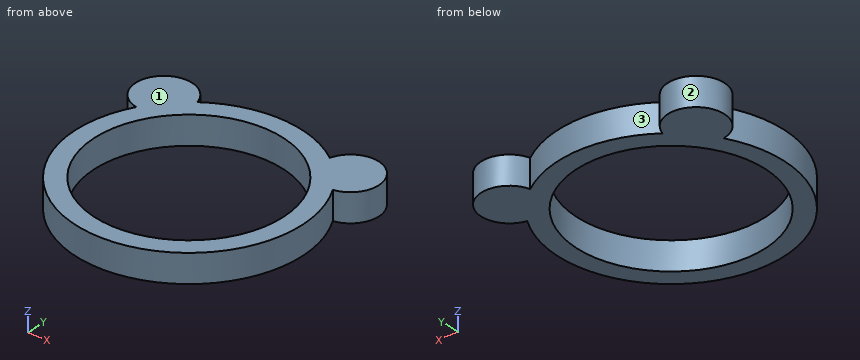
from build123d import *

# Parameters (mm, degrees)
CYLINDER002_R               = 10
CYLINDER002_DEPTH           = 10
CYLINDER001_R               = 3
CYLINDER001_DEPTH           = 3
CYLINDER001_PLACEMENT_ANGLE = 45
CYLINDER_R                  = 12
CYLINDER_DEPTH              = 3


with BuildPart() as hole:
    # Cylinder002 → Cylinder002 (new body)
    with BuildSketch(Plane.XY.offset(-4)):
        Circle(CYLINDER002_R)
    extrude(amount=CYLINDER002_DEPTH)


with BuildPart() as left_ear:
    # Cylinder001 → Cylinder001 (new body)
    with BuildSketch(Plane.XY):
        Circle(CYLINDER001_R)
    extrude(amount=CYLINDER001_DEPTH)


with BuildPart() as left_ear_1:
    # Cylinder001 placement: moved
    add(left_ear.part.moved(Location((-9.899495, 8.899495, 0))).rotate(Axis((-9.899495, 8.899495, 0), (0, 0, 1)), CYLINDER001_PLACEMENT_ANGLE))


with BuildPart() as right_ear:
    # Part__Mirroring: instance of left-ear
    add(left_ear_1.part.mirror(Plane(origin=(0, 0, 0), x_dir=(0, -1, 0), z_dir=(1, 0, 0))))


with BuildPart() as base_cylinder:
    # Cylinder → Cylinder (new body)
    with BuildSketch(Plane.XY):
        Circle(CYLINDER_R)
    extrude(amount=CYLINDER_DEPTH)


with BuildPart() as ring_with_ears:
    # Fusion base: copy of left-ear
    add(left_ear_1.part)

    # Fusion: union right-ear, base-cylinder
    add(right_ear.part)
    add(base_cylinder.part)

    # Cut: cut hole
    add(hole.part, mode=Mode.SUBTRACT)


solid = ring_with_ears.part
Source: CAD feature listing. Evaluate the final solid. Frame: model axes, mm. Face numbers are marked on the shaded views. Give positions to 0.01 mm unless a question says otherwise; leave off trailing zeros. Write each loop counter-clockwise with the first axis right and the second up, starting at its lowest first coordinate (ties: lowest second). Pieces come first, ordered by that corner, then holes. Notation, with made-up numbers: M 33,-20 L 92,-20 A7 cw 92,-16 Z; hole C 13,29 d6. An arc over 180 degrees is marked long. Return JSON: item names as keys, results as strings. Group by question number.
1) Pull-direction query (X, two-part tool) for the marked faces 1, 2 and 3; classes: pulls with the +X half, pulls with the -X half, needs draft (parallel to the pull), parting line crosses it, or undercut.
2) Cut plane A-A, the plane y = 0. Output: boundary loops of the cut face in (x, z), plus the area to 3 significant figures.
3) Cut plane C-C, the plane z = 0.35. Output: boundary loops of the cut face in (x, y), plus the area to 3 significant figures.
4) Pin query (flat end, axial travel): P1, Ø1.5, axis at x = 9, z = 1.5, coming from the +Y side; P2, Ø1, axis at y = 6, z = 2.5, coming from the +X side; P3, Ø12, axis at x = -2.5, y = 6.5, coming from the +Z side. Return the tip coordinate at first contact, or that it passes through.
5) Material intervals for line 1 along X through (y, z) = (0, 1); line 2 along X through (y, z) = (-5.75, 2.6), sorted ascending. Write a range as [from, to].
Recorded:
{
 "1": {"face 1": "needs draft", "face 2": "undercut", "face 3": "undercut"},
 "2": {"outline": "M -12,0 L -10,0 L -10,3 L -12,3 Z; M 10,0 L 12,0 L 12,3 L 10,3 Z", "area": "12.0 mm²"},
 "3": {"outline": "M -10.42,5.95 A12 ccw long 10.42,5.95 A3 ccw long 7.02,9.73 A12 ccw -7.02,9.73 A3 ccw long Z; hole C 0,0 d20", "area": "183 mm²"},
 "4": {"P1": "stops at y = 11.9", "P2": "stops at x = 11.7", "P3": "stops at z = 3"},
 "5": {"line 1": "x = [-12, -10], [10, 12]", "line 2": "x = [-10.53, -8.18], [8.18, 10.53]"}
}
